```python
from build123d import *

# Parameters (mm, degrees)
RESSALTO_EXTRUS_O1_DEPTH = 5.6
ESBO_O1_3_W              = 12.1
ESBO_O1_3_H              = 15.6
ESBO_O1_3_H_2            = 2
RESSALTO_EXTRUS_O2_DEPTH = 2
RESSALTO_EXTRUS_O3_DEPTH = 1
RESSALTO_EXTRUS_O3_DRAFT = 30


with BuildPart() as part:
    # Esbo_o1 → Ressalto-extrus_o1 (new body)
    with BuildSketch(Plane.XY):
        Polygon((0, 0), (0, -2), (2, -2), (2, 17.6), (-14.1, 17.6), (-14.1, -2), (-12.1, -2), (-12.1, 0), (-12.1, 15.6), (0, 15.6), align=None)
    extrude(amount=RESSALTO_EXTRUS_O1_DEPTH)

    # Esbo_o1_3 → Ressalto-extrus_o2 (add)
    with BuildSketch(Plane.XY):
        Polygon((0, 0), (0, -2), (2, -2), (2, 17.6), (-14.1, 17.6), (-14.1, -2), (-12.1, -2), (-12.1, 0), (-12.1, 15.6), (0, 15.6), align=None)
        with Locations((-6.05, 7.8)):
            Rectangle(ESBO_O1_3_W, ESBO_O1_3_H)
        with Locations((-6.05, -1)):
            Rectangle(ESBO_O1_3_W, ESBO_O1_3_H_2)
    extrude(amount=-RESSALTO_EXTRUS_O2_DEPTH)


with BuildPart() as ressalto_extrus_o3_tool:
    # Esbo_o2 → Ressalto-extrus_o3 (with draft: the straight prism first)
    with BuildSketch(Plane.XY.offset(5.6)):
        Polygon((-11.1, -2), (-11.1, 14.6), (-1, 14.6), (-1, -2), (2, -2), (2, 17.6), (-14.1, 17.6), (-14.1, -2), align=None)
    extrude(amount=RESSALTO_EXTRUS_O3_DEPTH)
    # Ressalto-extrus_o3: the draft: its side faces are tilted about the plane it starts from
    ressalto_extrus_o3_sides = [ressalto_extrus_o3_tool.faces().sort_by_distance(p)[0] for p in [
        (-6.05, 17.6, 6.1),
        (-14.1, 7.8, 6.1),
        (-12.6, -2, 6.1),
        (-11.1, 6.3, 6.1),
        (-6.05, 14.6, 6.1),
        (-1, 6.3, 6.1),
        (0.5, -2, 6.1),
        (2, 7.8, 6.1),
    ]]
    draft(ressalto_extrus_o3_sides, Plane.XY.offset(5.6), RESSALTO_EXTRUS_O3_DRAFT)


with BuildPart() as part_1:
    add(part.part)

    # Ressalto-extrus_o3: add ressalto_extrus_o3_tool
    add(ressalto_extrus_o3_tool.part)


solid = part_1.part
```
Check sheet for the modelled part. Datum: model origin and axes. Units: mm. A direction names the side the tool comes from. Round coordinates to 2 decimals unless told otherwise and drop trailing zeros. Order: outer loops, then holes, each group sorted by start corner. A loop starts at its lowest first (then second) coordinate and runs counter-clockwise, first axis right, second up. Notation, with made-up numbers: M 66,-19.5 L 97,-19.5 A20 cw 97,-0.5 Z; hole C -2,32 d7. An arc over 180 degrees is marked long. Answer in a Markdown table with one row per item.
(1) Section check A-A on x = -8.25. Record the boundary of the cut face in (y, z).
Findings:
| item | result |
|---|---|
| outline | M -2,-2 L 17.6,-2 L 17.6,5.6 L 17.02,6.6 L 15.18,6.6 L 14.6,5.6 L 15.6,5.6 L 15.6,0 L -2,0 Z |
(2) Draft check along Z on faces 1 (the flat face through (-12.1, 7, 3)), 2 (the flat face through (-6, 17.6, 2)), 3 (the flat face through (-13.815, 7.937, 6.093)). Enter one of: +Z half, -Z half, draft (parallel to the pull), parting line (faces both ways), or undercut.
Findings:
| item | result |
|---|---|
| face 1 | undercut |
| face 2 | draft |
| face 3 | +Z half |
(3) Material ranges on line 1 along X through (y, z) = (2.75, 2.5); line 2 along Z through (x, y) = (-8.25, 3.5); line 3 along Y through (x, z) = (-9.75, 4), recorded low to high. Write a range as from..to.
Findings:
| item | result |
|---|---|
| line 1 | x = -14.1..-12.1, 0..2 |
| line 2 | z = -2..0 |
| line 3 | y = 15.6..17.6 |
(4) Gauge pin test, flat ends, axial feed: pin 1 (4.5 mm diameter, centred on x = -4.5, z = 2.5, fed in from -Y); pin 2 (3.5 mm diameter, centred on x = -4.5, y = 10.5, fed in from +Z). Record the tip position at first contact, or that the pin passes through.
Findings:
| item | result |
|---|---|
| pin 1 | stops at y = 15.6 |
| pin 2 | stops at z = 0 |
(5) Section check D-D on z = 6. Record the boundary of the cut face in (x, y), plus the area to 3 significant figures.
Findings:
| item | result |
|---|---|
| outline | M -13.87,-1.77 L -11.33,-1.77 L -11.33,14.83 L -0.77,14.83 L -0.77,-1.77 L 1.77,-1.77 L 1.77,17.37 L -13.87,17.37 Z |
| area | 124 mm^2 |
(6) Section check C-C on y = -0.25. Record the boundary of the cut face in (x, z), plus the area to 3 significant figures.
Findings:
| item | result |
|---|---|
| outline | M -14.1,-2 L 2,-2 L 2,5.6 L 1.42,6.6 L -0.42,6.6 L -1,5.6 L 0,5.6 L 0,0 L -12.1,0 L -12.1,5.6 L -11.1,5.6 L -11.68,6.6 L -13.52,6.6 L -14.1,5.6 Z |
| area | 59.4 mm^2 |
(7) Section check B-B on z = 3. Record the boundary of the cut face in (x, y), plus the area to 3 significant figures.
Findings:
| item | result |
|---|---|
| outline | M -14.1,-2 L -12.1,-2 L -12.1,15.6 L 0,15.6 L 0,-2 L 2,-2 L 2,17.6 L -14.1,17.6 Z |
| area | 103 mm^2 |
(8) Set-up check for faces 4 (the flat face through (-14.1, 8, 2)), 5 (the flat face through (0, 7, 3)), 6 (the flat face through (-11.385, 6.468, 6.093)): record each of +Z, -Z, +X, -X, +Y, -Y from which the full face is reachable in a straight line by a thin tool's end or side.
Findings:
| item | result |
|---|---|
| face 4 | +Z, -Z, -X, +Y, -Y |
| face 5 | -Y |
| face 6 | +Z, -Y |
